Geometry check sheet. Reference: the model listing, model coordinates, mm. A direction names the side the tool comes from. Give positions to 0.01 mm unless a question says otherwise; leave off trailing zeros. Loops run counter-clockwise (first coordinate to the right, second up) from the corner with the lowest first, then second, coordinate; pieces in that order, holes last.
1. Cross-section at A-A, the plane x = -5. Record the cut outline in (y, z), plus the area to 3 significant figures.
2. Cross-section at C-C, the plane z = 24. Record the cut outline in (x, y).
3. Tool access check on faces 4 (the cylindrical face through (-18, 0, 24)), 5 (the flat face through (-21.617, -7.479, 1.078)), 6 (the flat face through (-21, -6, 25)), 7 (the flat face through (-2, -0.08, -5.75)). Record the directions out of +Z, -Z, +X, -X, +Y, -Y that give a thin tool (end or side, any length) a straight path to the whole face; none if there is none.
4. Cross-section at D-D, the plane y = -10.25. Record the cut outline in (x, z).
5. Material ranges on L1, parallel to Z at x = -5, y = -0.5; L2, parallel to Y at x = -5, z = -2; L3, parallel to Z at x = -12, y = 3.75, recorded low to high.
6. Go/stop test with flat-tipped pins: pin 1 Ø4 at (x, z) = (-21, 21) entering from +Y; pin 2 Ø3 at (x, y) = (-33, -3) entering from -Z; pin 3 Ø8 at (y, z) = (4, -6) entering from +X; pin 4 Ø6 at (x, y) = (-16.5, 1.5) entering from -Z. Record where each tip stops, or that it passes through.
7. Release check for a two-part mould opening along X. For faces 1 (the flat face through (-30.282, -6.986, 4.27)), 2 (the flat face through (-14, -13, -1)), 3 (the cylindrical face through (-6.19, 0.08, -5.46)) record: +X half, -X half, draft (parallel to the pull), parting line (faces both ways), or undercut.
8. Cross-section at B-B, the plane y = -0.25. Record the cut outline in (x, z), plus the area to 3 significant figures.
from build123d import *

# Parameters (mm, degrees)
F0_R        = 1.5
F1_DEPTH    = 6
F3_DEPTH    = 3
F5_DEPTH    = 4
F6_R        = 8
F7_T1_DEPTH = 37.0000029882


# Not quite as in the source:
# - a fillet or chamfer that OpenCascade refuses, or shapes differently, is made with other operations: its cross-section is extruded or revolved along the edge and cut away or added


with BuildPart() as f1:
    # F0 (on Front) → F1 (new body, symmetric)
    with BuildSketch(Plane.XZ):
        with BuildLine():
            ThreePointArc((-28.3348189516, 9.855862975), (-17.3828091911, 24.4507248282), (0, 30))
            Line((0, 30), (0, 42))
            ThreePointArc((0, 42), (-29.0229029625, 30.3590366057), (-41.9574939735, 1.8891001728))
            Line((-41.9574939735, 1.8891001728), (-3.94234519, -11.3339275806))
            Line((-3.94234519, -11.3339275806), (0, 0))
            Line((0, 0), (-28.3348189516, 9.855862975))
        make_face()
        with Locations((-5, -4.5450530015)):
            Circle(F0_R, mode=Mode.SUBTRACT)
    extrude(amount=F1_DEPTH, both=True)

    # F2 (on face) → F3 (join)
    with BuildSketch(Plane.XZ.offset(6)):
        Polygon((-19.6181767132, 6.8239031926), (-28.3348189516, 9.855862975), (-32.2851626761, -1.4752824294), (-23.5605219032, -4.5100243881), align=None)
    extrude(amount=F3_DEPTH)

    # F4 (on face) → F5 (join)
    with BuildSketch(Plane.XZ.offset(9)):
        Polygon((0, 0), (-28.3348189516, 9.855862975), (-32.2851626761, -1.4752824294), (-3.9770946697, -11.4338295597), align=None)
    extrude(amount=F5_DEPTH)

    # F6
    f6_edges = [f1.edges().sort_by_distance(p)[0] for p in [
        (-41.957494, 0, 1.8891),
    ]]
    fillet(f6_edges, radius=F6_R)

    # F7: fillet of radius 5 on 1 edges, made by hand

    # F7_s2 → F7_t1 (cut)
    with BuildSketch(Plane(origin=(4.1079708061, 0, 11.783282106), x_dir=(0, 1, 0), z_dir=(-0.3291952284, 0, -0.9442618819))):
        with BuildLine():
            ThreePointArc((-8, -29.9999925295), (-11.5355339059, -28.5355264354), (-13, -24.9999925295))
            Line((-13, -24.9999925295), (-13, -29.9999925295))
            Line((-13, -29.9999925295), (-8, -29.9999925295))
        make_face()
    extrude(amount=F7_T1_DEPTH, mode=Mode.SUBTRACT)


solid = f1.part
Result:
1. outline: (-13, -11.07) - (-9, -11.07) - (-9, 1.74) - (-13, 1.74) - close; (-6, -10.97) - (6, -10.97) - (6, -6.05) - (-6, -6.05) - close; (-6, -3.05) - (6, -3.05) - (6, 1.74) - (-6, 1.74) - close; (-6, 29.58) - (6, 29.58) - (6, 41.7) - (-6, 41.7) - close
1. area: 313 mm2
2. outline: (-34.47, -6) - (-18, -6) - (-18, 6) - (-34.47, 6) - close
3. face 4: +X, +Y, -Y
3. face 5: -Z, +X
3. face 6: +Z, -X, -Y
3. face 7: -Z, +X, +Y, -Y
4. outline: (-31.78, -1.65) - (-3.98, -11.43) - (0, 0) - (-27.83, 9.68) - close
5. L1: z = -10.97 to -6.05, -3.05 to 1.74, 29.58 to 41.7
5. L2: y = -13 to -9, -6 to 6
5. L3: z = -8.53 to 4.17, 27.5 to 40.25
6. pin 1: stops at y = 6
6. pin 2: stops at z = -1.75
6. pin 3: stops at x = -0.7
6. pin 4: stops at z = -8.01
7. face 1: -X half
7. face 2: draft
7. face 3: undercut
8. outline: (-41.02, 9.04) arc R8 ccw to (-35.83, -0.24) - (-3.94, -11.33) - (0, 0) - (-28.33, 9.86) arc R30 cw to (0, 30) - (0, 42) arc R42 ccw to start; hole circle Ø3 at (-5, -4.55)
8. area: 1,020 mm2
